Autodesk Inventor part; units mm, degrees
ref_plane "Work Plane6" through (0, 20.4, 0) normal (0, -1, 0) x (1, 0, 0)
ref_plane "Work Plane7" through (0, 20.75, 0) normal (0, -1, 0) x (1, 0, 0)
ref_plane "Work Plane8" through (0, 26.3, 0) normal (0, 1, 0) x (1, 0, 0)
sketch "Sketch1" plane through (0, 0, 0) normal (1, 0, 0) x (0, 1, 0)
  line L0 (20.75, 2.1) -> (20.75, 1.7)
  line L1 (20.4, 1.6) -> (20.4, 0)
  line L2 (31, 0) -> (20.4, 0)
  line L3 (23.4, 7.5) -> (20.4, 7.5)
  line L4 (20.4, 7.5) -> (20.4, 2.2)
  line L5 (20.75, 1.95) -> (20.75, 1.7)
  line L6 (20.75, 1.7) -> (20.75, 1.65)
  line L7 (20.4, 2.2) -> (20.4, 2.15)
  line L8 (20.75, 1.65) -> (20.75, 1.6)
  line L9 (20.75, 1.6) -> (20.4, 1.6)
  line L10 (20.4, 2.15) -> (20.4, 2.1)
  line L11 (20.4, 2.1) -> (20.75, 2.1)
  line L12 (31, 0) -> (32, 0)
  line L13 (32, 0) -> (32, 2.45)
  line L14 (32, 2.45) -> (30.5, 2.45)
  line L15 (30.5, 2.45) -> (30.5, 2.125)
  line L16 (30.5, 2.125) -> (29.7, 2.125)
  line L17 (29.7, 2.125) -> (29.7, 2.45)
  line L18 (29.7, 2.45) -> (26.7, 2.45)
  line L19 (26.7, 2.45) -> (26.7, 2.125)
  line L20 (26.7, 2.125) -> (25.9, 2.125)
  line L21 (25.9, 2.125) -> (25.9, 2.45)
  line L22 (25.9, 2.45) -> (24.4, 2.45)
  line L23 (23.4, 2.5) -> (24.4, 2.5)
  line L24 (24.4, 2.5) -> (24.4, 2.45)
  line L25 (23.4, 2.5) -> (23.4, 7.5)
  line L26 (32, 2.45) -> (31, 2.45)
  line L27 (32, 2.45) -> (32, 1.45)
  point P0 (0, 0)
  dimension "d305" = 3
  dimension "d306" = 5.3
  dimension "d326" = 0.05
  dimension "d329" = 1.6
  dimension "d330" = 0.5
  dimension "d331" = 0.35
  dimension "d344" = 1
  dimension "d345" = 1.5
  dimension "d346" = 0.325
  dimension "d347" = 0.8
  dimension "d348" = 3
  dimension "d349" = 0.325
  dimension "d350" = 0.8
  dimension "d351" = 2.45
  dimension "d353" = 1
  dimension "d354" = 1
  dimension "d355" = 1
revolve "Revolution1" add sketch "Sketch1" angle 360 about axis through (0, 31, 0) along (0, -1, 0)
sketch "Sketch11" plane through (0, 20.4, 0) normal (0, -1, 0) x (1, 0, 0)
  line L0 (0, 0) -> (0, -5)
  line L1 (0, 0) -> (-5, 0)
  line L2 (0, 0) -> (0, 5)
  line L3 (0, 0) -> (5, 0)
  dimension "d309" = 5
  dimension "d310" = 5
  dimension "d311" = 5
  dimension "d312" = 5
hole "Hole9" at (0, 20.4, -5) at (-5, 20.4, 0) at (0, 20.4, 5) at (5, 20.4, 0) direction (0, 1, 0) diameter 1.9 depth 2 tip angle 118
chamfer "Chamfer6" distance 0.5 angle 45 2 edges at (0, 23.4, -7.5) (0, 20.4, -7.5)
sketch "Sketch12" plane through (0, 20.4, 0) normal (0, -1, 0) x (1, 0, 0)
  circle A0 centre (0, 0) radius 0.9439
  line L0 (0, 0) -> (-21.4854, 21.4854)
  line L1 (0, 0) -> (30.3849, 0) construction
  dimension "d324" = 135
ref_plane "Work Plane6" through (0, 20.4, 0) normal (0, -1, 0) x (1, 0, 0)
ref_plane "Work Plane7" through (0, 20.75, 0) normal (0, -1, 0) x (1, 0, 0)
thread "Thread17"
thread "Thread18"
thread "Thread19"
thread "Thread20"
chamfer "Chamfer8" distance 1 angle 45 1 edges at (0, 32, -2.45)
sketch "Sketch13" plane through (0, 32, 0) normal (0, 1, 0) x (1, 0, 0)
  circle A0 centre (0, 0) radius 1
  dimension "d359" = 2
hole "Hole10" at (0, 32, 0) direction (0, -1, 0) diameter 2 end through all
ref_plane "Work Plane8" through (0, 26.3, 0) normal (0, 1, 0) x (1, 0, 0)
ref_plane "Work Plane9" through (0, 30.1, 0) normal (0, 1, 0) x (1, 0, 0)
properties part number "None_Magnet_Extender_Split_Top" material "Aluminum 6061"
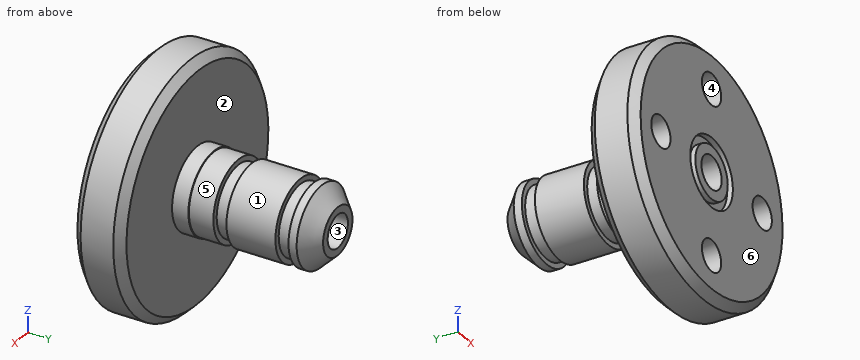
Verification items for the finished model (mm, model axes). Face numbers are marked on the shaded views. A direction names the side the tool comes from. Round coordinates to 2 decimals unless told otherwise and drop trailing zeros. Loops run counter-clockwise (first coordinate to the right, second up) from the corner with the lowest first, then second, coordinate; pieces in that order, holes last. Notation, with made-up numbers: (83, 8) -> (132, 8) arc R10 cw to (132, 18) -> close; hole circle Ø7 at (-24, 41). An arc over 180 degrees is marked (long way). Answer as a JSON object with one key per item and string values.
Q1. Go/stop test with flat-tipped pins: P1, Ø4, axis at y = 22.5, z = -5.5, coming from the -X side; P2, Ø1.5, axis at x = 0, z = 5, coming from the +Y side; P3, Ø1.1, axis at x = -5, z = 0, coming from the -Y side. Record where each tip stops, or that it passes through.
Data:
{"P1": "stops at x = -6.63", "P2": "stops at y = 23.4", "P3": "stops at y = 22.64"}
Q2. Scan lines: line 1 (Z direction, x = 0, y = 21); line 2 (X direction, y = 20.65, z = 0); line 3 (X direction, y = 26, z = 0) (3 decimals). Record each from-to range of solid material in increasing order. Write a range as from..to.
Data:
{"line 1": "z = -7.5..-5.95, -4.05..-1, 1..4.05, 5.95..7.5", "line 2": "x = -7.25..-5.95, -4.05..-2.1, -1.6..-1, 1..1.6, 2.1..4.05, 5.95..7.25", "line 3": "x = -2.125..-1, 1..2.125"}
Q3. Section check A-A (y = 30). Record the boundary of the cut face in (x, z) (3 decimals).
Data:
{"outline": "circle Ø4.25 at (0, 0); hole circle Ø2 at (0, 0)"}
Q4. Draft check along X on the marked faces 1, 2 and 3. Enter one of: pulls with the +X half, pulls with the -X half, needs draft (parallel to the pull), parting line crosses it, or undercut.
Data:
{"face 1": "parting line crosses it", "face 2": "needs draft", "face 3": "undercut"}
Q5. Access from +Z, -Z, +X, -X, +Y, -Y to the whole of each face (thin tool, end or side, straight path). Record for the marked faces 4, 5 and 6.
Data:
{"face 4": "-Y", "face 5": "+Y", "face 6": "+Z, -Z, +X, -X, -Y"}
